Design review of the part built by this model. Coordinates are the model's own, in mm. A direction names the side the tool comes from. Coordinates: 2 decimals unless noted, no trailing zeros. Loops run counter-clockwise (first coordinate to the right, second up) from the corner with the lowest first, then second, coordinate; pieces in that order, holes last.
Q1. Add section A-A on x = 0. Give the boundary of the cut face in (y, z), and give its area (3 significant figures).
Q2. Draft analysis for pull direction Y (two halves, no side actions). For faces 1 (the face through (-7.81, 6.245, 15.804)), 2 (the face through (-8.764, -1.987, 31.014)), 3 (the face through (-9.64, 2.25, 15.8)), state which applies: released by +Y, released by -Y, zero draft, split by the parting line, or undercut.
Q3. Wall thickness on probe 1 along Y at (x, z) = (0, 1.65); probe 2 along X at (y, z) = (0.25, 30); probe 3 along Y at (x, z) = (-1.75, 4): over which ranges is each line inside the solid? List them lowest first.
Q4. Add section B-B on z = 5.5. Give the boundary of the cut face in (x, y).
Q5. For P1, Ø5, axis at x = -7, z = 20.5, coming from the +Y side; P2, Ø6, axis at x = 3, y = -3, coming from the -Z side; P3, Ø1.5, axis at x = -5.5, z = 16, coming from the -Y side; P4, Ø4, axis at x = 0, y = -5.5, coming from the -Z side, all flat-tipped, find the tip position at first contact; note any pin that passes through.
Q6. Machinability: for faces 4 (the face through (7.71, -6.21, 15.8)), 5 (the face through (9.663, 2.154, 15.804)), 6 (the face through (0, 10, 16)), 7 (the face through (7.83, 6.22, 15.8)), which of the approach directions +Z, -Z, +X, -X, +Y, -Y give a long, thin tool a straight path to every point of the face, cutting with its end or side? Answer none if there is none.
```python
from build123d import *

# Parameters (mm, degrees)
AUFSATZ_LINEAR_AUSTRAGEN1_DEPTH      = 32
SKIZZE2_R                            = 11
AUFSATZ_LINEAR_AUSTRAGEN2_DEPTH      = 2
FASE1_SIZE                           = 2
SKIZZE3_R                            = 2.25
SCHNITT_LINEAR_AUSTRAGEN1_DEPTH      = 31.0000001
SCHNITT_LINEAR_AUSTRAGEN1_DEPTH_BACK = 3


with BuildPart() as part:
    # Skizze1 → Aufsatz-Linear austragen1 (new body)
    with BuildSketch(Plane.XY):
        with BuildLine():
            ThreePointArc((9.810830179, -1.325749297), (9.651786331, 2.202957246), (8.264031498, 5.451218525))
            ThreePointArc((8.264031498, 5.451218525), (7.818314825, 6.234898019), (7.153465102, 6.843824737))
            ThreePointArc((7.153465102, 6.843824737), (4.295449017, 8.919591792), (0.8906051, 9.859859155))
            ThreePointArc((0.8906051, 9.859859155), (0, 10), (-0.8906051, 9.859859155))
            ThreePointArc((-0.8906051, 9.859859155), (-4.295449017, 8.919591792), (-7.153465102, 6.843824737))
            ThreePointArc((-7.153465102, 6.843824737), (-7.818314825, 6.234898019), (-8.264031498, 5.451218525))
            ThreePointArc((-8.264031498, 5.451218525), (-9.651786331, 2.202957246), (-9.810830179, -1.325749297))
            ThreePointArc((-9.810830179, -1.325749297), (-9.749279122, -2.22520934), (-9.414473622, -3.062300839))
            ThreePointArc((-9.414473622, -3.062300839), (-7.740131676, -6.172549038), (-5.080440026, -8.497007069))
            ThreePointArc((-5.080440026, -8.497007069), (-4.338837391, -9.009688679), (-3.475625088, -9.269845212))
            ThreePointArc((-3.475625088, -9.269845212), (0, -9.9), (3.475625088, -9.269845212))
            ThreePointArc((3.475625088, -9.269845212), (4.338837391, -9.009688679), (5.080440026, -8.497007069))
            ThreePointArc((5.080440026, -8.497007069), (7.740131676, -6.172549038), (9.414473622, -3.062300839))
            ThreePointArc((9.414473622, -3.062300839), (9.749279122, -2.22520934), (9.810830179, -1.325749297))
        make_face()
    extrude(amount=AUFSATZ_LINEAR_AUSTRAGEN1_DEPTH)

    # Skizze2 → Aufsatz-Linear austragen2 (add)
    with BuildSketch(Plane.XY):
        Circle(SKIZZE2_R)
    extrude(amount=AUFSATZ_LINEAR_AUSTRAGEN2_DEPTH)

    # Fase1
    fase1_edges = [part.edges().sort_by_distance(p)[0] for p in [
        (7.818314825, 6.234898019, 32),
        (4.295449017, 8.919591792, 32),
        (0, 10, 32),
        (-4.295449017, 8.919591792, 32),
        (-7.818314825, 6.234898019, 32),
        (-9.651786331, 2.202957246, 32),
        (-9.749279122, -2.22520934, 32),
        (-7.740131676, -6.172549038, 32),
        (-4.338837391, -9.009688679, 32),
        (0, -9.9, 32),
        (9.651786331, 2.202957246, 32),
        (4.338837391, -9.009688679, 32),
        (7.740131676, -6.172549038, 32),
        (9.749279122, -2.22520934, 32),
    ]]
    chamfer(fase1_edges, length=FASE1_SIZE)

    # Skizze3 → Schnitt-Linear austragen1 (cut, two sides)
    with BuildSketch(Plane.XY.offset(2)) as schnitt_linear_austragen1_sk:
        with Locations((0, 5.5)):
            Circle(SKIZZE3_R)
        with Locations((5.5, 0)):
            Circle(SKIZZE3_R)
        with Locations((0, -5.5)):
            Circle(SKIZZE3_R)
        with Locations((-5.5, 0)):
            Circle(SKIZZE3_R)
    extrude(amount=SCHNITT_LINEAR_AUSTRAGEN1_DEPTH, mode=Mode.SUBTRACT)
    extrude(schnitt_linear_austragen1_sk.sketch, amount=-SCHNITT_LINEAR_AUSTRAGEN1_DEPTH_BACK, mode=Mode.SUBTRACT)


solid = part.part
```
Entries:
1. outline: (-11, 0) - (-7.75, 0) - (-7.75, 32) - (-7.9, 32) - (-9.9, 30) - (-9.9, 2) - (-11, 2) - close; (-3.25, 0) - (3.25, 0) - (3.25, 32) - (-3.25, 32) - close; (7.75, 0) - (11, 0) - (11, 2) - (10, 2) - (10, 30) - (8, 32) - (7.75, 32) - close
1. area: 349 mm2
2. face 1: released by +Y
2. face 2: undercut
2. face 3: split by the parting line
3. probe 1: y = -11 to -7.75, -3.25 to 3.25, 7.75 to 11
3. probe 2: x = -9.9 to -7.74, -3.26 to 3.26, 7.74 to 9.9
3. probe 3: y = -9.74 to -6.91, -4.09 to 4.09, 6.91 to 9.74
4. outline: (-9.81, -1.33) arc R2.9 ccw to (-9.41, -3.06) arc R9.9 ccw to (-5.08, -8.5) arc R2.9 ccw to (-3.48, -9.27) arc R9.9 ccw to (3.48, -9.27) arc R2.9 ccw to (5.08, -8.5) arc R9.9 ccw to (9.41, -3.06) arc R2.9 ccw to (9.81, -1.33) arc R9.9 ccw to (8.26, 5.45) arc R2.9 ccw to (7.15, 6.84) arc R9.9 ccw to (0.89, 9.86) arc R2.9 ccw to (-0.89, 9.86) arc R9.9 ccw to (-7.15, 6.84) arc R2.9 ccw to (-8.26, 5.45) arc R9.9 ccw to start; hole circle Ø4.5 at (-5.5, 0); hole circle Ø4.5 at (0, -5.5); hole circle Ø4.5 at (0, 5.5); hole circle Ø4.5 at (5.5, 0)
5. P1: stops at y = 8.82
5. P2: stops at z = 0
5. P3: stops at y = -8.77
5. P4: passes through
6. face 4: +Z, +X, -Y
6. face 5: +Z, +X
6. face 6: +Z, +Y
6. face 7: +Z, +X, +Y
